Can you work these out from the model? Positions are in its coordinate system, mm. A direction names the side the tool comes from. Give positions to 0.01 mm unless a question says otherwise; leave off trailing zeros. Write each loop counter-clockwise with the first axis right and the second up, starting at its lowest first coordinate (ties: lowest second). Pieces come first, ordered by that corner, then holes.
```python
from build123d import *

# Parameters (mm, degrees)
ESQUISSE1_R        = 1
BOSS_EXTRU_1_DEPTH = 40
ESQUISSE2_R        = 1.5
BOSS_EXTRU_2_DEPTH = 1


with BuildPart() as part:
    # Esquisse1 → Boss.-Extru.1 (new body)
    with BuildSketch(Plane.XY):
        Circle(ESQUISSE1_R)
    extrude(amount=BOSS_EXTRU_1_DEPTH)

    # Esquisse2 → Boss.-Extru.2 (add)
    with BuildSketch(Plane.XY.offset(40)):
        Circle(ESQUISSE2_R)
    boss_extru_2 = extrude(amount=BOSS_EXTRU_2_DEPTH)

    # Symétrie1: Boss.-Extru.2 across plane
    add(boss_extru_2.mirror(Plane(origin=(0, 0, 20), x_dir=(1, 0, 0), z_dir=(0, 0, -1))))


solid = part.part
```
1) Please list where these lines run through material, in increasing order: L1, parallel to Z at x = -0.65, y = -1.15; L2, parallel to Y at x = -0.05, z = 25.5; L3, parallel to Y at x = -0.45, z = 28.
Values follow:
L1: z = -1 to 0, 40 to 41
L2: y = -1 to 1
L3: y = -0.89 to 0.89
2) For faces 1 (the face through (0, 0, 41)), 2 (the face through (0, -1, 20)), which set-ups out of +Z, -Z, +X, -X, +Y, -Y let a thin tool reach every point of the face, with its end or its side?
Values follow:
face 1: +Z, +X, -X, +Y, -Y
face 2: none
3) Suppose I cut it at A-A on x = 0. Write out the boundary of the cut face in (y, z).
Values follow:
outline: (-1.5, -1) - (1.5, -1) - (1.5, 0) - (1, 0) - (1, 40) - (1.5, 40) - (1.5, 41) - (-1.5, 41) - (-1.5, 40) - (-1, 40) - (-1, 0) - (-1.5, 0) - close
4) For pin 1 Ø1.5 at (y, z) = (0, 17.5) entering from +X; pin 2 Ø1 at (y, z) = (-1, 26.5) entering from -X, each with a flat end and sliding along its axis, tell me the tip position at first contact or that it passes through.
Values follow:
pin 1: stops at x = 1
pin 2: stops at x = -0.87
5) Suppose I cut it at C-C on z = 19. Write out the boundary of the cut face in (x, y).
Values follow:
outline: circle Ø2 at (0, 0)
